Design review of the part built by this model. Coordinates are the model's own, in mm. A direction names the side the tool comes from. Round coordinates to 2 decimals unless told otherwise and drop trailing zeros. Order: outer loops, then holes, each group sorted by start corner. A loop starts at its lowest first (then second) coordinate and runs counter-clockwise, first axis right, second up. Notation, with made-up numbers: (-23.75, 29) - (35.25, 29) arc R18 cw to (35.25, 58) - close; hole circle Ø11 at (79.5, -22). An arc over 180 degrees is marked (long way). Write item = value, one per line.
Autodesk Inventor part; units mm, degrees
ref_plane "YZ Plane" through (0, 0, 0) normal (1, 0, 0) x (0, 1, 0)
ref_plane "XZ Plane" through (0, 0, 0) normal (0, 1, 0) x (-1, 0, 0)
ref_plane "XY Plane" through (0, 0, 0) normal (0, 0, 1) x (1, 0, 0)
sketch "草图1" plane through (0, 0, 0) normal (0, 0, 1) x (1, 0, 0)
  line L0 (80, -42.5) -> (-80, -42.5)
  line L1 (-80, 42.5) -> (80, 42.5)
  line L2 (80, -42.5) -> (-80, 42.5) construction
  line L3 (-80, -42.5) -> (80, 42.5) construction
  arc A0 (-80, 42.5) -> (-80, -42.5) centre (-45.0894, 0) ccw
  line L4 (0, 50.4113) -> (0, -46.1071) construction
  line L5 (96.3853, 0) -> (-113.3157, 0) construction
  line L6 (0, 24) -> (80, 24) construction
  line L7 (-155.9274, 0) -> (142.3547, 0) construction
  arc A1 (80, 24) -> (80, -24) centre (99.7429, 0) ccw
  arc A2 (80, 24) -> (80, 42.5) centre (75.8823, 33.25) ccw
  arc A3 (80, -42.5) -> (80, -24) centre (75.8823, -33.25) ccw
  circle A4 centre (0, 0) radius 7.5
  line L8 (0, 0) -> (-30.1738, 30.1738) construction
  arc A5 (-21.2132, 21.2132) -> (-20.0583, 22.3084) centre (0, 0) ccw construction
  arc A6 (-11.6701, 9.4239) -> (-9.4239, 11.6701) centre (0, 0) ccw construction
  line L9 (-10.6066, 10.6066) -> (-11.738, 9.4752) construction
  circle A7 centre (0, 0) radius 22.5 construction
  line L10 (-20.0818, 22.3446) -> (-9.4752, 11.738)
  line L11 (-10.6066, 10.6066) -> (-11.738, 9.4752) construction
  line L12 (-11.738, 9.4752) -> (-22.3446, 20.0818)
  line L13 (-20.0818, 22.3446) -> (-11.738, 9.4752) construction
  line L14 (-9.4752, 11.738) -> (-22.3446, 20.0818) construction
  arc A8 (-20.0818, 22.3446) -> (-22.3446, 20.0818) centre (-21.0865, 21.0865) ccw
  line L15 (-15.9099, 15.9099) -> (-9.5106, 22.3092) construction
  arc A9 (-11.738, 9.4752) -> (-9.4752, 11.738) centre (-10.7333, 10.7333) ccw
  line L16 (-24.1102, -7.5) -> (-24.1102, 7.5)
  line L17 (-20.9102, 7.4054) -> (-20.9102, -7.4054)
  line L18 (-20.9102, -7.4054) -> (-24.1102, 7.5) construction
  line L19 (-24.1102, -7.5) -> (-20.9102, 7.4054) construction
  arc A10 (-20.9102, 7.4054) -> (-24.1102, 7.5) centre (-22.5153, 7.28) ccw
  arc A11 (-24.1102, -7.5) -> (-20.9102, -7.4054) centre (-22.5153, -7.28) ccw
  line L20 (-31.8198, 0) -> (-31.8198, 22) construction
  line L21 (-31.8198, 22) -> (-64.8198, 22) construction
  line L22 (-31.8198, 22) -> (-31.8198, 33) construction
  line L23 (-31.8198, 33) -> (-64.8198, 33) construction
  line L24 (-39.9788, -4.6927) -> (-61.0474, -4.6927)
  line L25 (-62.4271, 5.3073) -> (-38.5991, 5.3073)
  line L26 (-39.9788, -4.6927) -> (-62.4271, 5.3073) construction
  line L27 (-61.0474, -4.6927) -> (-38.5991, 5.3073) construction
  arc A12 (-62.4271, 5.3073) -> (-61.0474, -4.6927) centre (-60.2132, 0.5176) ccw
  line L28 (-50.5131, 0) -> (-50.5131, 11.6306) construction
  arc A13 (-39.9788, -4.6927) -> (-38.5991, 5.3073) centre (-40.813, 0.5176) ccw
  line L29 (22.3446, 20.0818) -> (11.738, 9.4752)
  line L30 (9.4752, 11.738) -> (20.0818, 22.3446)
  arc A14 (22.3446, 20.0818) -> (20.0818, 22.3446) centre (21.0865, 21.0865) ccw
  arc A15 (9.4752, 11.738) -> (11.738, 9.4752) centre (10.7333, 10.7333) ccw
  line L31 (7.4054, 20.9102) -> (-7.4054, 20.9102)
  line L32 (-7.5, 24.1102) -> (7.5, 24.1102)
  arc A16 (7.4054, 20.9102) -> (7.5, 24.1102) centre (7.28, 22.5153) ccw
  arc A17 (-7.5, 24.1102) -> (-7.4054, 20.9102) centre (-7.28, 22.5153) ccw
  line L33 (20.0818, -22.3446) -> (9.4752, -11.738)
  line L34 (11.738, -9.4752) -> (22.3446, -20.0818)
  arc A18 (20.0818, -22.3446) -> (22.3446, -20.0818) centre (21.0865, -21.0865) ccw
  arc A19 (11.738, -9.4752) -> (9.4752, -11.738) centre (10.7333, -10.7333) ccw
  line L35 (20.9102, -7.4054) -> (20.9102, 7.4054)
  line L36 (24.1102, 7.5) -> (24.1102, -7.5)
  arc A20 (20.9102, -7.4054) -> (24.1102, -7.5) centre (22.5153, -7.28) ccw
  arc A21 (24.1102, 7.5) -> (20.9102, 7.4054) centre (22.5153, 7.28) ccw
  line L37 (-22.3446, -20.0818) -> (-11.738, -9.4752)
  line L38 (-9.4752, -11.738) -> (-20.0818, -22.3446)
  arc A22 (-22.3446, -20.0818) -> (-20.0818, -22.3446) centre (-21.0865, -21.0865) ccw
  arc A23 (-9.4752, -11.738) -> (-11.738, -9.4752) centre (-10.7333, -10.7333) ccw
  line L39 (-7.4054, -20.9102) -> (7.4054, -20.9102)
  line L40 (7.5, -24.1102) -> (-7.5, -24.1102)
  arc A24 (-7.4054, -20.9102) -> (-7.5, -24.1102) centre (-7.28, -22.5153) ccw
  arc A25 (7.5, -24.1102) -> (7.4054, -20.9102) centre (7.28, -22.5153) ccw
  line L41 (39.9788, -4.6927) -> (61.0474, -4.6927)
  line L42 (62.4271, 5.3073) -> (38.5991, 5.3073)
  arc A26 (61.0474, -4.6927) -> (62.4271, 5.3073) centre (60.2132, 0.5176) ccw
  arc A27 (38.5991, 5.3073) -> (39.9788, -4.6927) centre (40.813, 0.5176) ccw
  point P0 (-22.5, 0)
  point P1 (78.044, 33.25)
  point P2 (78.044, -33.25)
  point P3 (-53.8198, 22)
  point P4 (-42.8198, 22)
  point P5 (-53.8198, 33)
  point P6 (-42.8198, 33)
  point P7 (-80, 0)
  point P8 (-80, 15)
  point P9 (-80, 30)
  point P10 (-31.8198, -22)
  point P11 (-64.8198, -22)
  point P12 (-53.8198, -22)
  point P13 (-42.8198, -22)
  point P14 (-31.8198, -33)
  point P15 (-64.8198, -33)
  point P16 (-53.8198, -33)
  point P17 (-42.8198, -33)
  point P18 (-80, -15)
  point P19 (-80, -30)
  point P20 (31.8198, 22)
  point P21 (64.8198, 22)
  point P22 (53.8198, 22)
  point P23 (42.8198, 22)
  point P24 (31.8198, 33)
  point P25 (64.8198, 33)
  point P26 (53.8198, 33)
  point P27 (42.8198, 33)
  point P28 (31.8198, -33)
  point P29 (31.8198, -22)
  point P30 (42.8198, -33)
  point P31 (42.8198, -22)
  point P32 (53.8198, -33)
  point P33 (53.8198, -22)
  point P34 (64.8198, -33)
  point P35 (64.8198, -22)
  point P36 (-91.0115, 7.5)
  point P37 (11.6701, 9.4239)
  point P38 (9.4239, 11.6701)
  point P39 (9.4239, -11.6701)
  point P40 (11.6701, -9.4239)
  point P41 (-11.6701, -9.4239)
  point P42 (-9.4239, -11.6701)
  point P43 (-91.0115, -7.5)
  dimension "d0" = 160
  dimension "d1" = 24
  dimension "d2" = 85
  dimension "d3" = 15
  dimension "d4" = 45
  dimension "d5" = 60
  dimension "d6" = 30
  dimension "d7" = 1.6
  dimension "d8" = 45
  dimension "d9" = 3.2
  dimension "d10" = 15
  dimension "d11" = 1.61
  dimension "d12" = 1.61
  dimension "d13" = 22
  dimension "d15" = 11
  dimension "d16" = 11
  dimension "d17" = 11
  dimension "d18" = 33
  dimension "d19" = 55
  dimension "d20" = 15
  dimension "d21" = 15
  dimension "d22" = 10
  dimension "d25" = 7.5
  dimension "d28" = 360
  dimension "d41" = 1.6
extrude "拉伸1" add sketch "草图1" along normal blind 4 contours L0 A0 L1 A2 A1 A3 | L29 A15 L30 A14 | L31 A17 L32 A16 | L33 A19 L34 A18 | L35 A21 L36 A20 | L37 A23 L38 A22 | L39 A25 L40 A24 | A27 L42 A26 L41
extrude "拉伸2" cut sketch "草图1" along normal through all contours L29 A15 L30 A14 | L31 A17 L32 A16 | L33 A19 L34 A18 | L35 A21 L36 A20 | L37 A23 L38 A22 | L39 A25 L40 A24
extrude "拉伸3" cut sketch "草图1" along normal through all contours A27 L42 A26 L41
hole "孔1" at (78.044, 33.25, 0) at (78.044, -33.25, 0) at (-31.8198, 22, 0) at (-64.8198, 22, 0) at (-53.8198, 22, 0) at (-42.8198, 22, 0) at (-31.8198, 33, 0) at (-64.8198, 33, 0) at (-53.8198, 33, 0) at (-42.8198, 33, 0) at (-80, 0, 0) at (-80, 15, 0) at (-80, 30, 0) at (-31.8198, -33, 0) at (-31.8198, -22, 0) at (-42.8198, -33, 0) at (-42.8198, -22, 0) at (-53.8198, -33, 0) at (-53.8198, -22, 0) at (-64.8198, -33, 0) at (-64.8198, -22, 0) at (-80, -30, 0) at (-80, -15, 0) at (42.8198, 22, 0) at (42.8198, 33, 0) at (53.8198, 33, 0) at (53.8198, 22, 0) at (64.8198, 22, 0) at (64.8198, -22, 0) at (53.8198, -22, 0) at (42.8198, -22, 0) at (31.8198, -22, 0) at (31.8198, -33, 0) at (42.8198, -33, 0) at (53.8198, -33, 0) at (64.8198, -33, 0) at (-91.0115, 7.5, 0) at (-91.0115, -7.5, 0) at (31.8198, 33, 0) at (31.8198, 22, 0) at (64.8198, 33, 0) direction (0, 0, 1) diameter 3.2 end through all
properties part number "底盘设计1.2" material "聚碳酸酯，透明"
1) We need section A-A on x = 48. Write out the cut boundary in (y, z).
Findings:
outline = (-42.5, 0) - (-4.69, 0) - (-4.69, 4) - (-42.5, 4) - close; (5.31, 0) - (42.5, 0) - (42.5, 4) - (5.31, 4) - close
2) We need section C-C on z = 1.6. Give the number of separate pieces and of enclosed holes in the cut face, and give its area (3 significant figures).
Findings:
separate_pieces = 1
enclosed_holes = 52
area = 13,100 mm^2
3) For faces 5 (the cylindrical face through (68.67, -0.38, 1.97)), 6 (the cylindrical face through (8.89, 22.5, 1.97)), list the 3-axis set-ups (+Z, -Z, +X, -X, +Y, -Y) from which the entire face can be reached by the end or side of a thin tool; tool diameter is ignored.
Findings:
face_5 = +Z, -Z, +X
face_6 = +Z, -Z
4) The part is to be moulded in two halves that separate along X. For faces 1 (the cylindrical face through (-8.888, 22.435, 1.972)), 2 (the cylindrical face through (86.006, 33.413, 1.972)), 3 (the cylindrical face through (-41.846, 31.73, 2.028)), 4 (the flat face through (-8, 1, 4)), say which applies: released by +X, released by -X, zero draft, split by the parting line, or undercut.
Findings:
face_1 = undercut
face_2 = released by +X
face_3 = undercut
face_4 = zero draft
5) We need section B-B on x = 15. Write out the cut boundary in (y, z), and give its area (3 significant figures).
Findings:
outline = (-42.5, 0) - (-17.26, 0) - (-17.26, 4) - (-42.5, 4) - close; (-12.74, 0) - (12.74, 0) - (12.74, 4) - (-12.74, 4) - close; (17.26, 0) - (42.5, 0) - (42.5, 4) - (17.26, 4) - close
area = 304 mm^2
6) To check wall thickness, follow L1, parallel to Y at x = -80, z = 1.7; L2, parallel to Y at x = -13, z = 3.6; L3, parallel to Y at x = 43, z = 2.75. State the ranges of each line that lie inside material, in increasing order. Write a range as from..to.
Findings:
L1 = -42.5..-31.6, -28.4..-16.6, -13.4..-1.6, 1.6..13.4, 16.6..28.4, 31.6..42.5
L2 = -42.5..-15.26, -10.74..10.74, 15.26..42.5
L3 = -42.5..-34.59, -31.41..-23.59, -20.41..-4.69, 5.31..20.41, 23.59..31.41, 34.59..42.5
7) Clearance check with flat-ended pins moving along their axes: pin 1 Ø1.9 at (x, y) = (-42.82, 33) entering from -Z; pin 2 Ø1.2 at (y, z) = (3, 1) entering from -X; pin 3 Ø1.5 at (y, z) = (15.5, 3.5) entering from +X; pin 4 Ø1 at (y, z) = (-24, 2) entering from -X. State where each tip first meets the part, or that it passes through.
Findings:
pin_1 = through
pin_2 = -100.04
pin_3 = 73.25
pin_4 = -94.82
